Input: dimensioned drawing with shaded views. Units: mm. Origin: part minimum x, y, z. A direction names the side the tool comes from. Give positions to 0.01 mm unless a question says otherwise; leave off trailing zeros. Order: outer loops, then holes, each group sorted by start corner. A loop starts at its lowest first (then second) coordinate and runs counter-clockwise, first axis right, second up. Notation, with made-up numbers: (65.5, 65.5) - (103.5, 65.5) arc R7 cw to (103.5, 76.5) - close; hole circle Ø6 at (-25.75, -31). An arc over 180 degrees is marked (long way). Use a Markdown table: item, result.
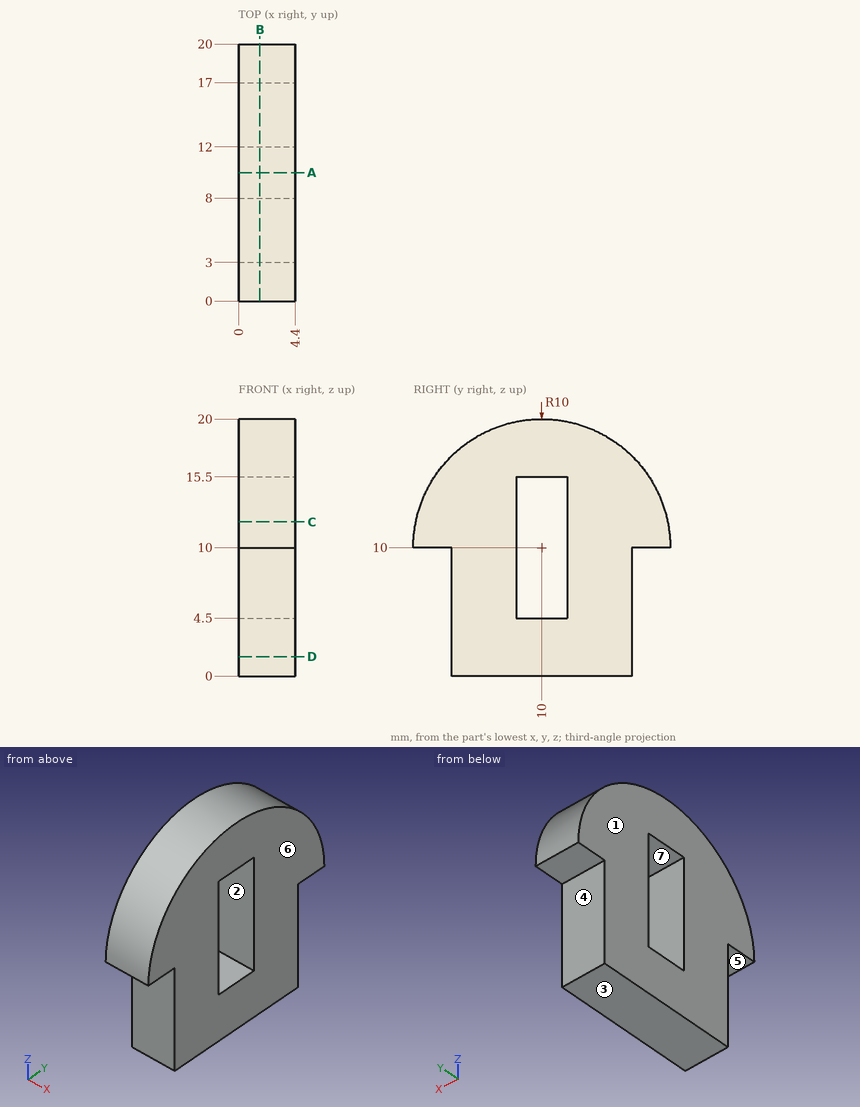
1. Section query B-B (x = 1.65). Return loops of the section in (y, z).
Response:
| item | result |
|---|---|
| outline | (0, 10) - (3, 10) - (3, 0) - (17, 0) - (17, 10) - (20, 10) arc R10 ccw to start; hole (8, 4.5) - (12, 4.5) - (12, 15.5) - (8, 15.5) - close |
2. Pin query (flat end, axial travel): pin 1 (2.5 mm diameter, centred on x = 1.5, y = 1, fed in from -Z); pin 2 (2 mm diameter, centred on x = 2, z = 3, fed in from -Y). Return the tip coordinate at first contact, or that it passes through.
Response:
| item | result |
|---|---|
| pin 1 | stops at z = 10 |
| pin 2 | stops at y = 3 |
3. Mould query, pull axis Z, two halves, no side actions, for the marked faces 1, 2 and 3. Classes: pulls with the +Z half, pulls with the -Z half, needs draft (parallel to the pull), parting line crosses it, or undercut.
Response:
| item | result |
|---|---|
| face 1 | needs draft |
| face 2 | undercut |
| face 3 | pulls with the -Z half |
4. Section query C-C (z = 12). Return loops of the section in (x, y).
Response:
| item | result |
|---|---|
| outline | (0, 0.2) - (4.4, 0.2) - (4.4, 8) - (0, 8) - close; (0, 12) - (4.4, 12) - (4.4, 19.8) - (0, 19.8) - close |
5. Set-up query: the marked faces 4, 5, 6 and 7. Return all of +Z, -Z, +X, -X, +Y, -Y with unobstructed straight access to the full face (end or side cutting, diameter ignored); none if empty.
Response:
| item | result |
|---|---|
| face 4 | -Z, +X, -X, +Y |
| face 5 | -Z, +X, -X, -Y |
| face 6 | +Z, -Z, +X, +Y, -Y |
| face 7 | +X, -X |
6. Section query A-A (y = 10). Return loops of the section in (x, z), then the cut area to 3 significant figures.
Response:
| item | result |
|---|---|
| outline | (0, 0) - (4.4, 0) - (4.4, 4.5) - (0, 4.5) - close; (0, 15.5) - (4.4, 15.5) - (4.4, 20) - (0, 20) - close |
| area | 39.6 mm^2 |
7. Section query D-D (z = 1.5). Return loops of the section in (x, y).
Response:
| item | result |
|---|---|
| outline | (0, 3) - (4.4, 3) - (4.4, 17) - (0, 17) - close |
8. Material intervals for line 1 along Y through (x, z) = (1.55, 4.75); line 2 along Y through (x, z) = (3.2, 10.25); line 3 along Z through (x, y) = (3.95, 10), sorted ascending.
Response:
| item | result |
|---|---|
| line 1 | y = 3 to 8, 12 to 17 |
| line 2 | y = 0 to 8, 12 to 20 |
| line 3 | z = 0 to 4.5, 15.5 to 20 |
